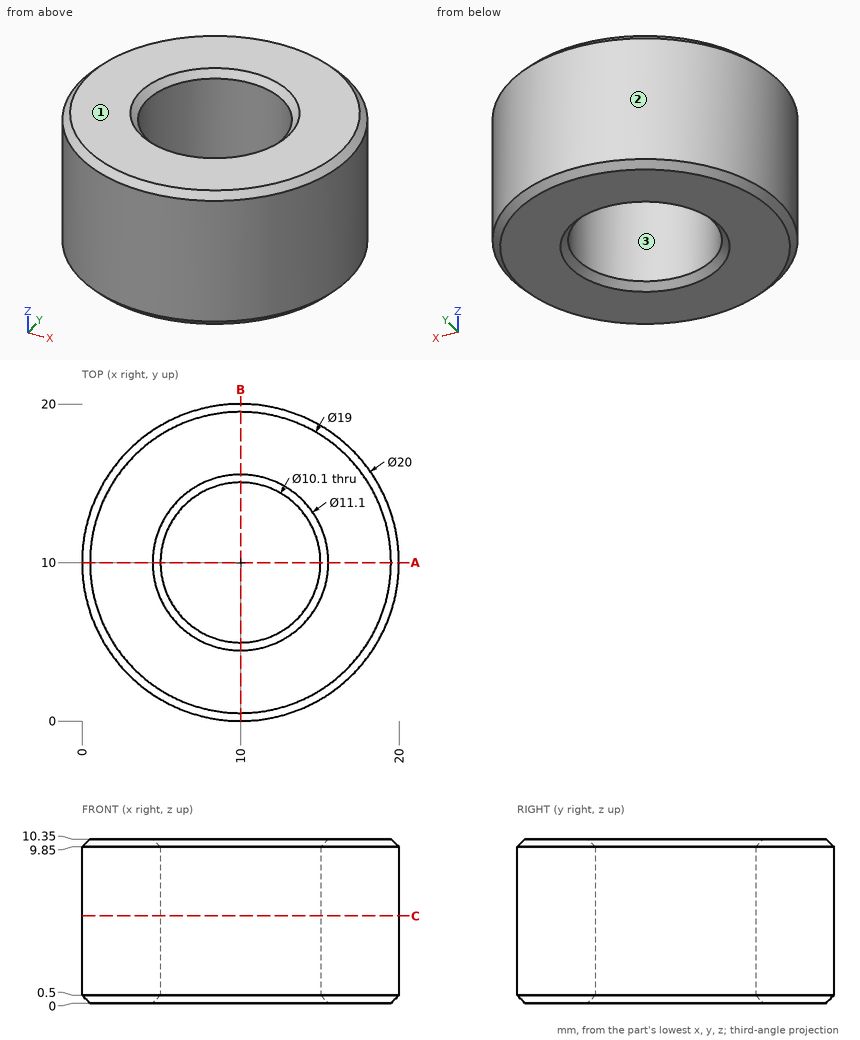
Design review of the part shown in the three views and the two pictorial views. Dimensions are in mm from the part's minimum x, y and z. Give positions to 0.01 mm unless a question says otherwise; leave off trailing zeros. Write each loop counter-clockwise with the first axis right and the second up, starting at its lowest first coordinate (ties: lowest second). Pieces come first, ordered by that corner, then holes. Notation, with made-up numbers: M 11.25,73 L 20.25,73 A11 cw 20.25,93 Z; hole C -16.75,22 d7. An arc over 180 degrees is marked long. Return JSON: item names as keys, results as strings. Group by question number.
Item 1: The part is to be moulded in two halves that separate along X. For the marked faces 1, 2 and 3, say which applies: pulls with the +X half, pulls with the -X half, needs draft (parallel to the pull), parting line crosses it, or undercut.
Item 2: Clearance check with flat-ended pins moving along their axes: pin 1 Ø2 at (x, z) = (17.5, 1) entering from +Y; pin 2 Ø6 at (x, y) = (10, 10) entering from -Z; pin 3 Ø1 at (x, z) = (8, 6.5) entering from -Y; pin 4 Ø1 at (x, z) = (6, 9) entering from -Y. State where each tip first meets the part, or that it passes through.
Item 3: Take a section at A-A (y = 10). Give the boundary of the cut face in (x, z), plus the area to 3 significant figures.
Item 4: Wall thickness on line 1 along Y through (x, z) = (10, 6.5); line 2 along X through (y, z) = (11.5, 5.5); line 3 along X through (y, z) = (6, 8.5): over which ranges is each line inside the solid? List them lowest first.
Item 5: Take a section at C-C (z = 5.5). Give the boundary of the cut face in (x, y), plus the area to 3 significant figures.
Return value:
{
 "1": {"face 1": "needs draft", "face 2": "parting line crosses it", "face 3": "undercut"},
 "2": {"pin 1": "stops at y = 17.6", "pin 2": "passes through", "pin 3": "stops at y = 0.11", "pin 4": "stops at y = 0.63"},
 "3": {"outline": "M 0,0.5 L 0.5,0 L 4.45,0 L 4.95,0.5 L 4.95,9.85 L 4.45,10.35 L 0.5,10.35 L 0,9.85 Z; M 15.05,0.5 L 15.55,0 L 19.5,0 L 20,0.5 L 20,9.85 L 19.5,10.35 L 15.55,10.35 L 15.05,9.85 Z", "area": "101 mm2"},
 "4": {"line 1": "y = 0 to 4.95, 15.05 to 20", "line 2": "x = 0.11 to 5.18, 14.82 to 19.89", "line 3": "x = 0.83 to 6.92, 13.08 to 19.17"},
 "5": {"outline": "C 10,10 d20; hole C 10,10 d10.1", "area": "234 mm2"}
}
